Input: part model. Units: mm. Frame: model coordinates. A direction names the side the tool comes from. Give positions to 0.01 mm unless a question says otherwise; leave off trailing zeros. Loops run counter-clockwise (first coordinate to the right, second up) from the corner with the lowest first, then second, coordinate; pieces in that order, holes last. Notation, with made-up numbers: (32.25, 36.5) - (89.25, 36.5) arc R8 ccw to (89.25, 51.5) - close; hole circle Ø3 at (-17.75, -12). An arc over 180 degrees is marked (long way). Answer as a JSON object with one key per item and string values. Group by question number.
(1) Section query D-D (y = 1.5). Return loops of the section in (x, z).
(2) Section query B-B (y = 8). Return loops of the section in (x, z), plus the area to 3 significant figures.
(3) Section query A-A (x = 15). Return loops of the section in (y, z).
(4) Pin query (flat end, axial travel): P1, Ø3.5, axis at x = 15, z = 3, coming from the -Y side; P2, Ø1.6, axis at y = 3, z = 7, coming from the +X side; P3, Ø4, axis at y = 1.5, z = -4, coming from the +X side. Return the tip coordinate at first contact, or that it passes through.
(5) Material intervals for L1, parallel to Z at x = -11.5, y = 3.75; L2, parallel to X at y = 8.4, z = 3; L3, parallel to Y at x = -3.5, z = 0.25, sorted ascending.
(6) Access query for faces 1 (the flat face through (-13, 0, 7)), 2 (the flat face through (10, 2, -7)), 3 (the flat face through (-25, 2, 0)). Directions: +Z, -Z, +X, -X, +Y, -Y. A direction counts if a zero-diameter tool reaches every point of the face in a straight line with its end or side. Return the directions, or none.
(7) Mould query, pull axis X, two halves, no side actions, for faces 4 (the cylindrical face through (16.265, 7.958, 2.194)), 5 (the flat face through (10, 2, 7)), 6 (the flat face through (0, 5, 0)). Classes: +X half, -X half, draft (parallel to the pull), parting line (faces both ways), or undercut.
(8) Section query C-C (x = -9.5). Return loops of the section in (y, z), plus the area to 3 significant figures.
```python
from build123d import *

# Parameters (mm, degrees)
BOSS_EXTRUDE1_DEPTH     = 5
BOSS_EXTRUDE2_DEPTH     = 6
SKETCH4_R               = 1.5
CUT_EXTRUDE1_DEPTH      = 29.806292715
CUT_EXTRUDE2_DEPTH      = 33.385336188
CUT_EXTRUDE2_DEPTH_BACK = 33.385336188
SKETCH5_W               = 15
SKETCH5_H               = 5


with BuildPart() as part:
    # Sketch2 → Boss-Extrude1 (new body)
    with BuildSketch(Plane(origin=(0, 0, 0), x_dir=(1, 0, 0), z_dir=(0, 1, 0))):
        Polygon((-27, 8.05), (25, 8.05), (25, 6.05), (-21.55, 6.05), (-25, 2.6), (-25, -2.6), (-21.55, -6.05), (25, -6.05), (25, -8.05), (-27, -8.05), align=None)
    extrude(amount=BOSS_EXTRUDE1_DEPTH)

    # Sketch3 → Boss-Extrude2 (add)
    with BuildSketch(Plane(origin=(0, 5, 0), x_dir=(1, 0, 0), z_dir=(0, 1, 0))):
        Polygon((25, 6.05), (25, -6.05), (25, -8.05), (-27, -8.05), (-27, 8.05), (25, 8.05), align=None)
    extrude(amount=BOSS_EXTRUDE2_DEPTH)

    # Sketch4 → Cut-Extrude1 (cut, through all)
    with BuildSketch(Plane.XZ.offset(-5)):
        with Locations(Location((15, 3, 0), (0, 0, 270))):
            Circle(SKETCH4_R)
        with Locations(Location((15, -3, 0), (0, 0, 270))):
            Circle(SKETCH4_R)
    extrude(amount=-CUT_EXTRUDE1_DEPTH, mode=Mode.SUBTRACT)

    # Sketch5 → Cut-Extrude2 (cut, two sides: drawn at the far end of the back side and taken through both)
    with BuildSketch(Plane(origin=(0, 0, 6.05), x_dir=(-1, 0, 0), z_dir=(0, 0, -1)).offset(-CUT_EXTRUDE2_DEPTH_BACK)):
        with Locations((-17.5, 2.5)):
            Rectangle(SKETCH5_W, SKETCH5_H)
    extrude(amount=CUT_EXTRUDE2_DEPTH + CUT_EXTRUDE2_DEPTH_BACK, mode=Mode.SUBTRACT)


solid = part.part
```
Recorded:
{
 "1": {"outline": "(-27, -8.05) - (10, -8.05) - (10, -6.05) - (-21.55, -6.05) - (-25, -2.6) - (-25, 2.6) - (-21.55, 6.05) - (10, 6.05) - (10, 8.05) - (-27, 8.05) - close"},
 "2": {"outline": "(-27, -8.05) - (25, -8.05) - (25, 8.05) - (-27, 8.05) - close; hole circle Ø3 at (15, -3); hole circle Ø3 at (15, 3)", "area": "823 mm^2"},
 "3": {"outline": "(5, -8.05) - (11, -8.05) - (11, -4.5) - (5, -4.5) - close; (5, -1.5) - (11, -1.5) - (11, 1.5) - (5, 1.5) - close; (5, 4.5) - (11, 4.5) - (11, 8.05) - (5, 8.05) - close"},
 "4": {"P1": "stops at y = 5", "P2": "stops at x = 10", "P3": "stops at x = -21.6"},
 "5": {"L1": "z = -8.05 to -6.05, 6.05 to 8.05", "L2": "x = -27 to 13.5, 16.5 to 25", "L3": "y = 5 to 11"},
 "6": {"face 1": "+Z, -Z, +X, -X, -Y", "face 2": "+Z, -Z, +X, -Y", "face 3": "+X, -Y"},
 "7": {"face 4": "undercut", "face 5": "+X half", "face 6": "draft"},
 "8": {"outline": "(0, -8.05) - (11, -8.05) - (11, 8.05) - (0, 8.05) - (0, 6.05) - (5, 6.05) - (5, -6.05) - (0, -6.05) - close", "area": "117 mm^2"}
}
